Verification items for the finished model (mm, model axes). A direction names the side the tool comes from. Round coordinates to 2 decimals unless told otherwise and drop trailing zeros. Write each loop counter-clockwise with the first axis right and the second up, starting at its lowest first coordinate (ties: lowest second). Pieces come first, ordered by that corner, then holes. Notation, with made-up numbers: M 12.5,-13.5 L 55.5,-13.5 A18 ccw 55.5,-5.5 Z; hole C -5,-3 d1. An arc over 180 degrees is marked long. One line per question, with ' | ' between items.
Autodesk Fusion 360 part; units mm, degrees
sketch "Sketch1" plane through (0, 0, 0) normal (0, 0, 1) x (1, 0, 0)
  line L0 (0, 0) -> (0, 50) construction
  line L1 (3, 50) -> (-3, 50)
  line L2 (-3, 50) -> (-3, 44)
  line L3 (-3, 44) -> (3, 44)
  line L4 (3, 44) -> (3, 50)
  line L5 (3, 50) -> (-3, 44) construction
  line L6 (-3, 50) -> (3, 44) construction
  line L7 (3, 3) -> (-3, 3)
  line L8 (-3, 3) -> (-3, -3)
  line L9 (-3, -3) -> (3, -3)
  line L10 (3, -3) -> (3, 3)
  line L11 (3, 3) -> (-3, -3) construction
  line L12 (-3, 3) -> (3, -3) construction
  line L13 (0.75, 44) -> (0.75, 3)
  line L14 (-0.75, 44) -> (-0.75, 3)
  line L15 (-50, -3) -> (-44, -3)
  line L16 (-50, 3) -> (-50, -3)
  line L17 (-44, 3) -> (-50, 3)
  line L18 (-44, -3) -> (-44, 3)
  line L19 (-44, -0.75) -> (-3, -0.75)
  line L20 (-44, 0.75) -> (-3, 0.75)
  line L21 (3, -50) -> (3, -44)
  line L22 (-3, -50) -> (3, -50)
  line L23 (-3, -44) -> (-3, -50)
  line L24 (3, -44) -> (-3, -44)
  line L25 (0.75, -44) -> (0.75, -3)
  line L26 (-0.75, -44) -> (-0.75, -3)
  line L27 (50, 3) -> (44, 3)
  line L28 (50, -3) -> (50, 3)
  line L29 (44, -3) -> (50, -3)
  line L30 (44, 3) -> (44, -3)
  line L31 (44, 0.75) -> (3, 0.75)
  line L32 (44, -0.75) -> (3, -0.75)
  line L33 (3, 25) -> (-3, 25)
  line L34 (-3, 25) -> (-3, 19)
  line L35 (3, 19) -> (3, 25)
  line L36 (-3, 19) -> (3, 19)
  line L37 (-19, 3) -> (-25, 3)
  line L38 (-25, 3) -> (-25, -3)
  line L39 (-25, -3) -> (-19, -3)
  line L40 (-19, -3) -> (-19, 3)
  line L41 (-3, -19) -> (-3, -25)
  line L42 (-3, -25) -> (3, -25)
  line L43 (3, -25) -> (3, -19)
  line L44 (3, -19) -> (-3, -19)
  line L45 (19, -3) -> (25, -3)
  line L46 (25, -3) -> (25, 3)
  line L47 (25, 3) -> (19, 3)
  line L48 (19, 3) -> (19, -3)
  point P0 (0, 47)
  dimension "d1" = 50
  dimension "d2" = 6
  dimension "d3" = 6
  dimension "d4" = 6
  dimension "d5" = 6
  dimension "d6" = 1.5
  dimension "d8" = 360
  dimension "d13" = 6
  dimension "d14" = 6
  dimension "d15" = 25
  dimension "d17" = 360
extrude "Extrude1" add sketch "Sketch1" along normal blind 2
extrude "Extrude2" add sketch "Sketch1" along normal blind 20 contours L7 L8 L9 L10
1. Tool access check on faces 1 (the face through (0, 27, 2)), 2 (the face through (-27, 0, 2)), 3 (the face through (0, -26, 2)). Record the directions out of +Z, -Z, +X, -X, +Y, -Y that give a thin tool (end or side, any length) a straight path to the whole face; none if there is none.
Results:
face 1: +Z, +X, -X, +Y | face 2: +Z, -X, +Y, -Y | face 3: +Z, +X, -X, -Y
2. Section check B-B, the plane y = -21. Record the cut outline in (x, z), then the cut area to 3 significant figures.
Results:
outline: M -3,0 L 3,0 L 3,2 L -3,2 Z | area: 12.0 mm2
3. Thickness scan on line 1 (Y direction, x = -2, z = 2.5); line 2 (Y direction, x = 9.5, z = 1.75). Record the ranges inside material, lowest first.
Results:
line 1: y = -3 to 3 | line 2: y = -0.75 to 0.75
4. Go/stop test with flat-tipped pins: P1, Ø1, axis at x = 22, z = 1, coming from the +Y side; P2, Ø8, axis at y = -30, z = 5.5, coming from the +X side; P3, Ø0.6, axis at y = 48, z = 0.5, coming from the +X side. Record where each tip stops, or that it passes through.
Results:
P1: stops at y = 3 | P2: stops at x = 0.75 | P3: stops at x = 3
5. Section check A-A, the plane x = -29. Record the cut outline in (y, z).
Results:
outline: M -0.75,0 L 0.75,0 L 0.75,2 L -0.75,2 Z
